Model file for the job. Use its own axes, mm. A direction names the side the tool comes from. Coordinates: 2 decimals unless noted, no trailing zeros. Loops run counter-clockwise (first coordinate to the right, second up) from the corner with the lowest first, then second, coordinate; pieces in that order, holes last. Notation, with made-up numbers: (70.25, 16.5) -> (101.25, 16.5) arc R21 cw to (101.25, 45.5) -> close; hole circle Ø11 at (66.25, 35.5). An arc over 180 degrees is marked (long way). Use one line per item in the form item = value.
```python
from build123d import *

# Parameters (mm, degrees)
BOX002_W        = 2
BOX002_H        = 1.5
BOX002_DEPTH    = 2
CHAMFER003_SIZE = 0.75
BOX_W           = 2
BOX_H           = 3.5
BOX_DEPTH       = 2
BOX001_W        = 2
BOX001_H        = 1.5
BOX001_DEPTH    = 9
CHAMFER004_SIZE = 0.5
CHAMFER005_SIZE = 1
CHAMFER006_SIZE = 0.5
CHAMFER007_SIZE = 0.4


with BuildPart() as chamfer003:
    # Box002 → Box002 (new body)
    with BuildSketch(Plane(origin=(-1, 18.25, 7), x_dir=(1, 0, 0), z_dir=(0, 0, 1))):
        with Locations((1, 0.75)):
            Rectangle(BOX002_W, BOX002_H)
    extrude(amount=BOX002_DEPTH)

    # Chamfer003
    chamfer003_edges = [chamfer003.edges().sort_by_distance(p)[0] for p in [
        (0, 18.25, 7),
        (0, 18.25, 9),
    ]]
    chamfer(chamfer003_edges, length=CHAMFER003_SIZE)


with BuildPart() as cube:
    # Box → Box (new body)
    with BuildSketch(Plane(origin=(-1, 17, 0), x_dir=(1, 0, 0), z_dir=(0, 0, 1))):
        with Locations((1, 1.75)):
            Rectangle(BOX_W, BOX_H)
    extrude(amount=BOX_DEPTH)


with BuildPart() as chamfer007:
    # Box001 → Box001 (new body)
    with BuildSketch(Plane(origin=(-1, 19, 0), x_dir=(1, 0, 0), z_dir=(0, 0, 1))):
        with Locations((1, 0.75)):
            Rectangle(BOX001_W, BOX001_H)
    extrude(amount=BOX001_DEPTH)

    # Chamfer004
    chamfer004_edges = [chamfer007.edges().sort_by_distance(p)[0] for p in [
        (0, 20.5, 9),
    ]]
    chamfer(chamfer004_edges, length=CHAMFER004_SIZE)

    # Fusion: union Chamfer003, Cube
    add(chamfer003.part)
    add(cube.part)

    # Chamfer005
    chamfer005_edges = [chamfer007.edges().sort_by_distance(p)[0] for p in [
        (0, 20.5, 0),
    ]]
    chamfer(chamfer005_edges, length=CHAMFER005_SIZE)

    # Chamfer006
    chamfer006_edges = [chamfer007.edges().sort_by_distance(p)[0] for p in [
        (0, 19, 2),
    ]]
    chamfer(chamfer006_edges, length=CHAMFER006_SIZE)

    # Chamfer007
    chamfer007_edges = [chamfer007.edges().sort_by_distance(p)[0] for p in [
        (-1, 17.75, 2),
        (-1, 18.75, 2.25),
        (-1, 19, 4.75),
        (-1, 18.625, 7.375),
        (-1, 18.25, 8),
        (-1, 18.625, 8.625),
        (-1, 19.5, 9),
        (-1, 20.25, 8.75),
        (-1, 20.5, 4.75),
        (-1, 20, 0.5),
        (-1, 18.25, 0),
        (1, 17.75, 2),
        (1, 18.75, 2.25),
        (1, 19, 4.75),
        (1, 18.25, 0),
        (1, 18.625, 7.375),
        (1, 20, 0.5),
        (1, 18.25, 8),
        (1, 20.5, 4.75),
        (1, 18.625, 8.625),
        (1, 20.25, 8.75),
        (1, 19.5, 9),
    ]]
    chamfer(chamfer007_edges, length=CHAMFER007_SIZE)


solid = chamfer007.part
```
Q1. Which spindle directions (+Z, -Z, +X, -X, +Y, -Y) get a long thin tool onto all of the face, cutting with end or side? Do faces 1 (the face through (-0.8, 18.82, 7.46)), 2 (the face through (0.803, 18.888, 2.101)), 3 (the face through (0, 18, 2)). Say none if no direction does.
Result:
face_1 = -X, -Y
face_2 = +X, -Y
face_3 = +X, -X, -Y
Q2. Pin check, flat tips, straight feed: pin 1 Ø1 at (x, y) = (0.5, 17.5) entering from +Z; pin 2 Ø1 at (y, z) = (18, 5.5) entering from +X. Stop position of each tip, or through.
Result:
pin_1 = 2
pin_2 = through
Q3. Band-saw the part on D-D, the plane y = 17.7. Write the cut outline in (x, z).
Result:
outline = (-1, 0.4) -> (-0.6, 0) -> (0.6, 0) -> (1, 0.4) -> (1, 1.6) -> (0.6, 2) -> (-0.6, 2) -> (-1, 1.6) -> close
Q4. Band-saw the part on B-B, the plane z = 5.25. Write the cut outline in (x, y).
Result:
outline = (-1, 19.4) -> (-0.6, 19) -> (0.6, 19) -> (1, 19.4) -> (1, 20.1) -> (0.6, 20.5) -> (-0.6, 20.5) -> (-1, 20.1) -> close
Q5. Wall check: line 1 along Z through (x, y) = (-0.35, 19.9); line 2 along Z through (x, y) = (-0.8, 18.6); line 3 along Z through (x, y) = (-0.5, 18.05). Give the ranges that are in metal, low to high.
Result:
line_1 = 0.4 to 9
line_2 = 0.2 to 1.82, 7.68 to 8.32
line_3 = 0 to 2
Q6. Mould opens along Z. For faces 4 (the face through (0, 19, 5)), 5 (the face through (-0.8, 18.76, 8.48)), 6 (the face through (0.803, 19.85, 0.636)) say: released by +Z, released by -Z, zero draft, split by the parting line, or undercut.
Result:
face_4 = undercut
face_5 = released by +Z
face_6 = released by -Z
Q7. Band-saw the part on A-A, the plane y = 18.8. Write the cut outline in (x, z).
Result:
outline = (-1, 0.4) -> (-0.6, 0) -> (0.6, 0) -> (1, 0.4) -> (1, 1.73) -> (0.6, 2.3) -> (-0.6, 2.3) -> (-1, 1.73) -> close; (-1, 7.77) -> (-0.6, 7.2) -> (0.6, 7.2) -> (1, 7.77) -> (1, 8.23) -> (0.6, 8.8) -> (-0.6, 8.8) -> (-1, 8.23) -> close
Q8. Band-saw the part on C-C, the plane x = 0.1. Write the cut outline in (y, z), and give its area (3 significant figures).
Result:
outline = (17, 0) -> (19.5, 0) -> (20.5, 1) -> (20.5, 8.5) -> (20, 9) -> (19, 9) -> (18.25, 8.25) -> (18.25, 7.75) -> (19, 7) -> (19, 2.5) -> (18.5, 2) -> (17, 2) -> close
area = 17.9 mm2
